Drawing for the job (mm, zero at the part's lowest x, y, z). Give positions to 0.01 mm unless a question says otherwise; leave off trailing zeros. Order: outer loops, then holes, each group sorted by start corner. A loop starts at its lowest first (then second) coordinate and runs counter-clockwise, first axis right, second up. Notation, with made-up numbers: (12.5, -32) - (61.5, -32) arc R21 cw to (61.5, -10) - close; hole circle Ø3 at (52.5, 78). An arc over 180 degrees is marked (long way). One line per item, written item: value.
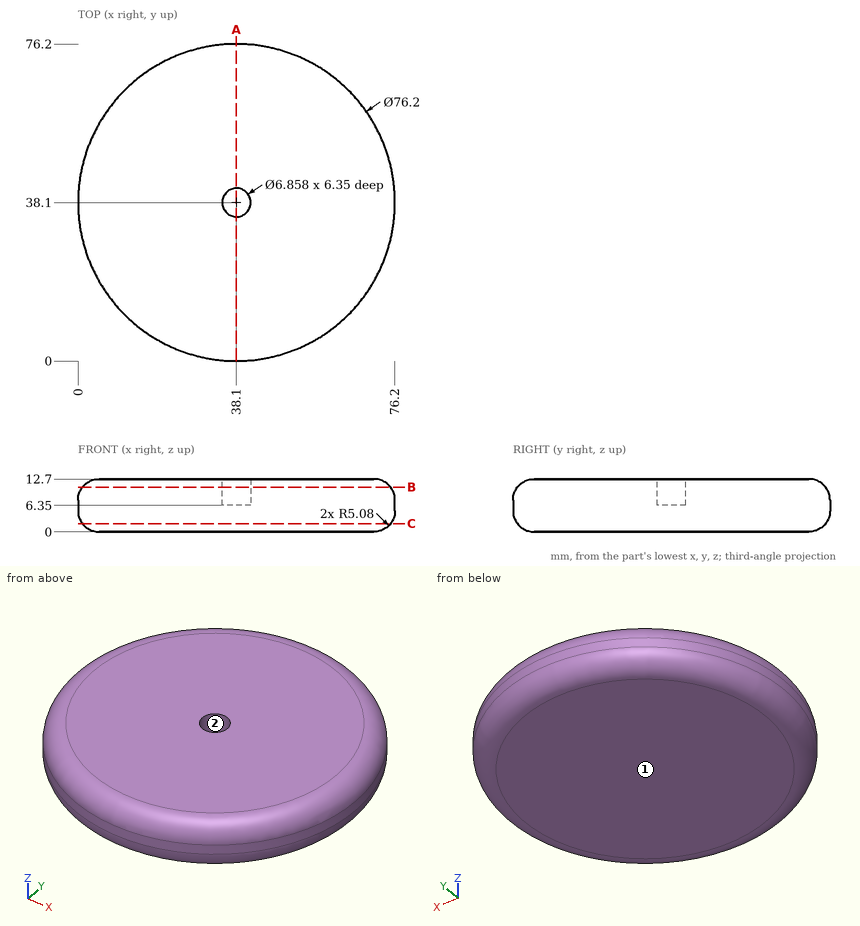
1) Cut at C-C, the plane z = 2. Give the cut face in (x, y).
Outcome:
outline: circle Ø74.12 at (38.1, 38.1)
2) Cut at B-B, the plane z = 10.75. Give the cut face in (x, y).
Outcome:
outline: circle Ø74.04 at (38.1, 38.1); hole circle Ø6.86 at (38.1, 38.1)
3) Drill centre lines: line 1 along Z through (x, y) = (52, 68.5); line 2 along Y through (x, z) = (38.1, 9.25); line 3 along X through (y, z) = (40, 9). Where is each one in solid material? Low to high. Write a range as from..to.
Outcome:
line 1: z = 0.02..12.68
line 2: y = 0.27..34.67, 41.53..75.93
line 3: x = 0.24..35.25, 40.95..75.96
4) Pin check, flat tips, straight feed: pin 1 (11 mm diameter, centred on x = 38.1, y = 38.1, fed in from -Z); pin 2 (2 mm diameter, centred on y = 33, z = 2, fed in from +X); pin 3 (4 mm diameter, centred on x = 25, z = 9, fed in from +Y); pin 4 (5 mm diameter, centred on x = 49.5, z = 8.5, fed in from -Y). Stop position of each tip, or through.
Outcome:
pin 1: stops at z = 0
pin 2: stops at x = 75.43
pin 3: stops at y = 74.46
pin 4: stops at y = 1.08
5) Mould opens along X. For the marked faces 1 and 2 say: released by +X, released by -X, zero draft, split by the parting line, or undercut.
Outcome:
face 1: zero draft
face 2: undercut
6) Cut at A-A, the plane x = 38.1. Give the cut face in (y, z).
Outcome:
outline: (0, 5.08) arc R5.08 ccw to (5.08, 0) - (71.12, 0) arc R5.08 ccw to (76.2, 5.08) - (76.2, 7.62) arc R5.08 ccw to (71.12, 12.7) - (41.53, 12.7) - (41.53, 6.35) - (34.67, 6.35) - (34.67, 12.7) - (5.08, 12.7) arc R5.08 ccw to (0, 7.62) - close
